Check sheet for the modelled part. Datum: model origin and axes. Units: mm. A direction names the side the tool comes from. Round coordinates to 2 decimals unless told otherwise and drop trailing zeros. Loops run counter-clockwise (first coordinate to the right, second up) from the corner with the lowest first, then second, coordinate; pieces in that order, holes last. Notation, with made-up numbers: (-30, -34) -> (18, -34) arc R15 ccw to (18, -30) -> close; hole circle Ø9 at (21.25, -18). An arc over 180 degrees is marked (long way). One line per item, written item: value. Start each with the question number.
1. Cross-section at B-B on x = -2.5. Record the cut outline in (y, z), then the cut area to 3 significant figures.
2. Cross-section at A-A on z = 6.5. Record the cut outline in (x, y), then the cut area to 3 significant figures.
3. Go/stop test with flat-tipped pins: pin 1 (4 mm diameter, centred on y = 24, z = 6, fed in from -X); pin 2 (5 mm diameter, centred on y = -10, z = 5.5, fed in from -X); pin 3 (2 mm diameter, centred on x = 21, z = 1.5, fed in from +Y). Record where each tip stops, or that it passes through.
4. Release check for a two-part mould opening along X. For faces 4 (the face through (47.493, -0.638, 5.493)), 5 (the face through (-1, 0, 0)), 6 (the face through (-17.5, -21, 5)) record: +X half, -X half, draft (parallel to the pull), parting line (faces both ways), or undercut.
5. Material ranges on L1, parallel to Y at x = -14.5, z = 3; L2, parallel to X at y = 21, z = 2.5; L3, parallel to X at y = -27, z = 0.5, recorded low to high.
6. Set-up check for faces 1 (the face through (0, 12.1, 5)), 2 (the face through (-47.493, 0.66, 5.493)), 3 (the face through (0, -12.1, 5)): record each of +Z, -Z, +X, -X, +Y, -Y from which the full face is reachable in a straight line by a thin tool's end or side.
from build123d import *

# Parameters (mm, degrees)
F0_W     = 35
F0_H     = 24.2
F1_DEPTH = 11.1
F2_R     = 1.5


with BuildPart() as f1:
    # F0 (on Top) → F1 (new body)
    with BuildSketch(Plane.XY):
        with BuildLine():
            Line((-17.5, -12.1), (-17.5, 12.1))
            Line((-17.5, 12.1), (-17.5, 30))
            ThreePointArc((-17.5, 30), (-47.5, 0), (-17.5, -30))
            Line((-17.5, -30), (-17.5, -12.1))
        make_face()
        with BuildLine():
            Line((17.5, 30), (17.5, 12.1))
            Line((17.5, 12.1), (17.5, -12.1))
            Line((17.5, -12.1), (17.5, -30))
            ThreePointArc((17.5, -30), (47.5, 0), (17.5, 30))
        make_face()
        Rectangle(F0_W, F0_H)
    extrude(amount=F1_DEPTH)

    # F2
    f2_edges = [f1.edges().sort_by_distance(p)[0] for p in [
        (-47.5, 0, 11.1),
        (-17.5, 21.05, 11.1),
        (-17.5, -21.05, 11.1),
        (0, -12.1, 11.1),
        (17.5, -21.05, 11.1),
        (47.5, 0, 11.1),
        (17.5, 21.05, 11.1),
        (0, 12.1, 11.1),
        (-17.5, -21.05, 0),
        (0, -12.1, 0),
        (17.5, -21.05, 0),
        (47.5, 0, 0),
        (17.5, 21.05, 0),
        (0, 12.1, 0),
        (-17.5, 21.05, 0),
        (-47.5, 0, 0),
        (17.5, -30, 5.55),
        (17.5, 30, 5.55),
    ]]
    fillet(f2_edges, radius=F2_R)


solid = f1.part
Taken from the geometry:
1. outline: (-12.1, 1.5) arc R1.5 ccw to (-10.6, 0) -> (10.6, 0) arc R1.5 ccw to (12.1, 1.5) -> (12.1, 9.6) arc R1.5 ccw to (10.6, 11.1) -> (-10.6, 11.1) arc R1.5 ccw to (-12.1, 9.6) -> close
1. area: 267 mm2
2. outline: (-17.5, -30) -> (-17.5, -12.1) -> (17.5, -12.1) -> (17.5, -28.46) arc R1.5 ccw to (19.08, -29.96) arc R30 ccw to (19.08, 29.96) arc R1.5 ccw to (17.5, 28.46) -> (17.5, 12.1) -> (-17.5, 12.1) -> (-17.5, 30) arc R30 ccw to start
2. area: 3,670 mm2
3. pin 1: stops at x = -37.9
3. pin 2: stops at x = -46.55
3. pin 3: stops at y = 29.9
4. face 4: +X half
4. face 5: draft
4. face 6: undercut
5. L1: y = -12.1 to 12.1
5. L2: x = -38.92 to -17.5, 17.5 to 38.92
5. L3: x = -29.67 to -17.88, 17.88 to 29.67
6. face 1: +Z, -Z, +Y
6. face 2: +Z, -Z, -X
6. face 3: +Z, -Z, -Y
